The listing builds one solid part. Answer for the finished solid, in the listing's coordinates (mm). A direction names the side the tool comes from. Coordinates: 2 decimals unless noted, no trailing zeros. Write each loop counter-clockwise with the first axis right and the second up, starting at its lowest first coordinate (ties: lowest second). Pieces come first, ordered by that corner, then holes.
(1) For a pull along X with two mould halves and no side action, classify faces 1 (the flat face through (-5.45, 0, 6)), 2 (the flat face through (-0.1, 6, 0.5)), 3 (the cylindrical face through (11.199, 5.715, 0.507)) as +X half, -X half, draft (parallel to the pull), parting line (faces both ways), or undercut.
(2) The part is cut by section A-A on z = 4. Determine the outline of the cut face in (x, y), plus the area to 3 significant figures.
(3) Which of the six approach directions +Z, -Z, +X, -X, +Y, -Y give full straight-line access (tool end or side, diameter ignored) to faces 4 (the flat face through (3.4, -5.3, 1)), 5 (the flat face through (-3.64, -0.06, 5.36)), 6 (the flat face through (-3, -4, 4)), 7 (the flat face through (-3, 4, 4))?
(4) Straight lines are drawn through the part: line 1 (X direction, y = 3, z = 4); line 2 (Z direction, x = -0.75, y = 2.25); line 3 (Z direction, x = 10, y = 3.75). For each, find the intervals that lie inside material, in ascending order.
(5) The part is cut by section D-D on z = 2.75. Determine the outline of the cut face in (x, y), plus the area to 3 significant figures.
(6) Given P1, Ø1, axis at y = -2, z = 5.5, coming from the -X side; P2, Ø1.2, axis at y = 2, z = 6, coming from the +X side; P3, Ø0.8, axis at y = 0.5, z = 6, coming from the -X side, each flat-ended and moving along its own axis, determine where each tip first touches the part or whether it passes through.
from build123d import *

# Parameters (mm, degrees)
SKETCH1_W           = 23
SKETCH1_H           = 12
BOSS_EXTRUDE1_DEPTH = 1
BOSS_EXTRUDE2_DEPTH = 4
LPATTERN2_COUNT     = 3
LPATTERN2_PITCH     = 6.5
FILLET1_R           = 1
FILLET2_R           = 1


with BuildPart() as part:
    # Sketch1 → Boss-Extrude1 (new body)
    with BuildSketch(Plane.XY):
        Rectangle(SKETCH1_W, SKETCH1_H)
    extrude(amount=BOSS_EXTRUDE1_DEPTH)

    # Sketch3 → Boss-Extrude2 (add, symmetric)
    with BuildSketch(Plane.XZ):
        with BuildLine():
            Line((-10.5, 1), (-10.5, 4.371779789))
            Line((-10.5, 4.371779789), (-9.772059531, 6.371779789))
            Line((-9.772059531, 6.371779789), (-9.05, 6.371779789))
            Line((-9.05, 6.371779789), (-9.05, 4.871779789))
            ThreePointArc((-9.05, 4.871779789), (-7.25, 2), (-5.45, 4.871779789))
            Line((-5.45, 4.871779789), (-5.45, 6.371779789))
            Line((-5.45, 6.371779789), (-4.727940469, 6.371779789))
            Line((-4.727940469, 6.371779789), (-4, 4.371779789))
            Line((-4, 4.371779789), (-4, 1))
            Line((-4, 1), (-10.5, 1))
        make_face()
    boss_extrude2 = extrude(amount=BOSS_EXTRUDE2_DEPTH, both=True)

    # LPattern2: Boss-Extrude2 ×3
    with Locations(*[(i * LPATTERN2_PITCH, 0, 0) for i in range(1, LPATTERN2_COUNT)]):
        add(boss_extrude2)

    # Fillet1
    fillet1_edges = [part.edges().sort_by_distance(p)[0] for p in [
        (-11.5, 6, 0.5),
        (11.5, 6, 0.5),
        (11.5, -6, 0.5),
        (-11.5, -6, 0.5),
    ]]
    fillet(fillet1_edges, radius=FILLET1_R)

    # Fillet2
    fillet2_edges = [part.edges().sort_by_distance(p)[0] for p in [
        (-0.75, 4, 1),
        (-10.5, 0, 1),
        (-0.75, -4, 1),
        (9, 0, 1),
    ]]
    fillet(fillet2_edges, radius=FILLET2_R - 0.0001)  # a hair under: the kernel refuses the full size


solid = part.part
Model answer:
1. face 1: undercut
1. face 2: draft
1. face 3: +X half
2. outline: (-10.5, -4) - (-9.25, -4) - (-9.25, 4) - (-10.5, 4) - close; (-5.25, -4) - (-2.75, -4) - (-2.75, 4) - (-5.25, 4) - close; (1.25, -4) - (3.75, -4) - (3.75, 4) - (1.25, 4) - close; (7.75, -4) - (9, -4) - (9, 4) - (7.75, 4) - close
2. area: 60.0 mm2
3. face 4: +Z, +X
3. face 5: +Z, +Y, -Y
3. face 6: +Z, +X, -X, -Y
3. face 7: +Z, +X, -X, +Y
4. line 1: x = -10.5 to -9.25, -5.25 to -2.75, 1.25 to 3.75, 7.75 to 9
4. line 2: z = 0 to 2
4. line 3: z = 0 to 1
5. outline: (-10.5, -4) - (-8.81, -4) - (-8.81, 4) - (-10.5, 4) - close; (-5.69, -4) - (-2.31, -4) - (-2.31, 4) - (-5.69, 4) - close; (0.81, -4) - (4.19, -4) - (4.19, 4) - (0.81, 4) - close; (7.31, -4) - (9, -4) - (9, 4) - (7.31, 4) - close
5. area: 81.1 mm2
6. P1: stops at x = -10.27
6. P2: stops at x = 8.63
6. P3: stops at x = -10.05
